For this review, take the finished solid that the model builds, in its own axes (mm). Give positions to 0.01 mm unless a question says otherwise; leave off trailing zeros. Write each loop counter-clockwise with the first axis right and the second up, starting at its lowest first coordinate (ties: lowest second). Pieces come first, ordered by that corner, then holes.
from build123d import *

# Parameters (mm, degrees)
CROQUIS1_W              = 55
CROQUIS1_H              = 55
CROQUIS1_R              = 20
CROQUIS1_R_2            = 3
CROQUIS1_R_3            = 1.5
SALIENTE_EXTRUIR1_DEPTH = 2
REDONDEO1_R             = 5


with BuildPart() as part:
    # Croquis1 → Saliente-Extruir1 (new body)
    with BuildSketch(Plane.XY):
        Rectangle(CROQUIS1_W, CROQUIS1_H)
        Circle(CROQUIS1_R, mode=Mode.SUBTRACT)
        with Locations((-22.550252532, 22.550252532)):
            Circle(CROQUIS1_R_2, mode=Mode.SUBTRACT)
        with Locations((22.550252532, 22.550252532)):
            Circle(CROQUIS1_R_2, mode=Mode.SUBTRACT)
        with Locations((22.550252532, -22.550252532)):
            Circle(CROQUIS1_R_2, mode=Mode.SUBTRACT)
        with Locations((-22.550252532, -22.550252532)):
            Circle(CROQUIS1_R_2, mode=Mode.SUBTRACT)
        with Locations((0, 23.5)):
            Circle(CROQUIS1_R_3, mode=Mode.SUBTRACT)
        with Locations((23.5, 0)):
            Circle(CROQUIS1_R_3, mode=Mode.SUBTRACT)
        with Locations((0, -23.5)):
            Circle(CROQUIS1_R_3, mode=Mode.SUBTRACT)
        with Locations((-23.5, 0)):
            Circle(CROQUIS1_R_3, mode=Mode.SUBTRACT)
    extrude(amount=SALIENTE_EXTRUIR1_DEPTH)

    # Redondeo1
    redondeo1_edges = [part.edges().sort_by_distance(p)[0] for p in [
        (-27.5, 27.5, 1),
        (27.5, 27.5, 1),
        (27.5, -27.5, 1),
        (-27.5, -27.5, 1),
    ]]
    fillet(redondeo1_edges, radius=REDONDEO1_R)


solid = part.part
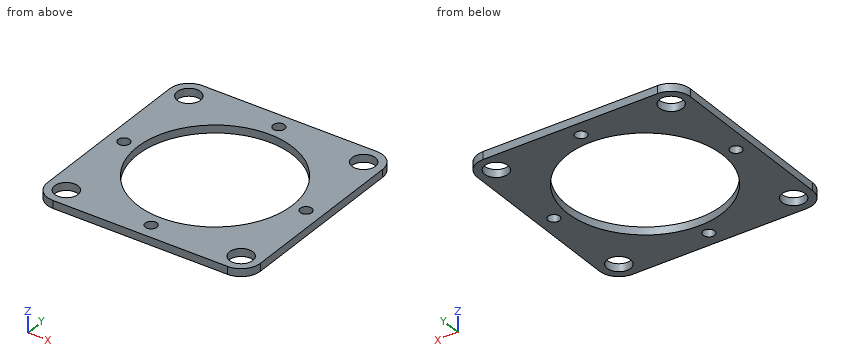
(1) We need section B-B (x = 16). Write out the cut boundary in (y, z).
(2) We need section A-A (y = 0). Write out the cut boundary in (x, z), and give its area (3 significant figures).
(3) Clearance check with a flat-ended pin moving along its axis: pin 1 Ø3.5 at (x, y) = (22.55, -22.55) entering from +Z. State where the tip first meets the part, or that it passes through.
(4) We need section D-D (y = -13). Write out the cut boundary in (x, z).
(5) For L1, parallel to Y at x = 0, z = 1.5; L2, parallel to Y at x = -23.5, z = 0.75; L3, parallel to Y at x = 20.5, z = 0.6, list the stretches that pass through material, from the lowest coordinate up.
The answers:
1. outline: (-27.5, 0) - (-12, 0) - (-12, 2) - (-27.5, 2) - close; (12, 0) - (27.5, 0) - (27.5, 2) - (12, 2) - close
2. outline: (-27.5, 0) - (-25, 0) - (-25, 2) - (-27.5, 2) - close; (-22, 0) - (-20, 0) - (-20, 2) - (-22, 2) - close; (20, 0) - (22, 0) - (22, 2) - (20, 2) - close; (25, 0) - (27.5, 0) - (27.5, 2) - (25, 2) - close
2. area: 18.0 mm2
3. pin 1: passes through
4. outline: (-27.5, 0) - (-15.2, 0) - (-15.2, 2) - (-27.5, 2) - close; (15.2, 0) - (27.5, 0) - (27.5, 2) - (15.2, 2) - close
5. L1: y = -27.5 to -25, -22 to -20, 20 to 22, 25 to 27.5
5. L2: y = -27.4 to -25.4, -19.7 to -1.5, 1.5 to 19.7, 25.4 to 27.4
5. L3: y = -27.5 to -24.74, -20.36 to 20.36, 24.74 to 27.5
